Input: dimensioned drawing with shaded views. Units: mm. Origin: part minimum x, y, z. A direction names the side the tool comes from. Coordinates: 2 decimals unless noted, no trailing zeros. Order: outer loops, then holes, each group sorted by start corner. A loop starts at its lowest first (then second) coordinate and runs counter-clockwise, first axis right, second up. Notation, with made-up numbers: (43.25, 83.5) -> (84.25, 83.5) arc R20 ccw to (84.25, 90.5) -> close; hole circle Ø8 at (-12, 13). An arc over 180 degrees is marked (long way). Answer as CSV lines item,"result".
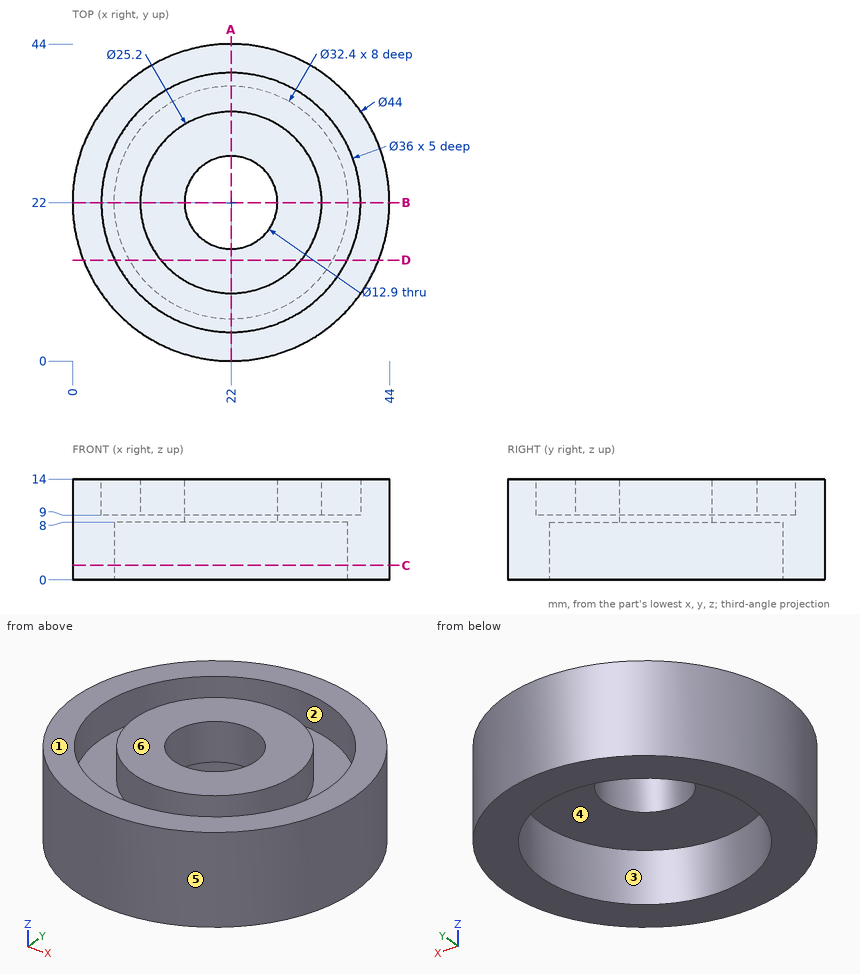
1. Ray query, line 1 along Y through (x, z) = (22, 11.5); line 2 along Y through (x, z) = (22, 6.25); line 3 along X through (y, z) = (13.5, 10.5). Return the intervals inside material, ascending.
Findings:
line 1,"y = 0 to 4, 9.4 to 15.55, 28.45 to 34.6, 40 to 44"
line 2,"y = 0 to 5.8, 38.2 to 44"
line 3,"x = 1.71 to 6.13, 12.7 to 31.3, 37.87 to 42.29"
2. Mould query, pull axis Y, two halves, no side actions, for the marked faces 4, 5 and 6. Classes: released by +Y, released by -Y, zero draft, split by the parting line, or undercut.
Findings:
face 4,"undercut"
face 5,"split by the parting line"
face 6,"zero draft"
3. Contact query for flat-ended pins moving along their axis: pin 1 (6 mm diameter, centred on x = 31.5, y = 31, fed in from +Z); pin 2 (4 mm diameter, centred on y = 34, z = 8.5, fed in from -X); pin 3 (16 mm diameter, centred on x = 22.5, y = 17.5, fed in from -Z); pin 4 (2 mm diameter, centred on x = 34, z = 3.5, fed in from -Y). Output: stop coordinate, or through.
Findings:
pin 1,"stops at z = 14"
pin 2,"stops at x = 2.4"
pin 3,"stops at z = 8"
pin 4,"stops at y = 2.95"
4. Cut plane C-C (z = 2). Return the cut outline in (x, y).
Findings:
outline,"circle Ø44 at (22, 22); hole circle Ø32.4 at (22, 22)"
5. Cut plane A-A (x = 22). Return the cut outline in (y, z), plus the area to 3 significant figures.
Findings:
outline,"(0, 0) -> (5.8, 0) -> (5.8, 8) -> (15.55, 8) -> (15.55, 14) -> (9.4, 14) -> (9.4, 9) -> (4, 9) -> (4, 14) -> (0, 14) -> close; (28.45, 8) -> (38.2, 8) -> (38.2, 0) -> (44, 0) -> (44, 14) -> (40, 14) -> (40, 9) -> (34.6, 9) -> (34.6, 14) -> (28.45, 14) -> close"
area,"225 mm2"
6. Cut plane D-D (y = 14). Return the cut outline in (x, z), plus the area to 3 significant figures.
Findings:
outline,"(1.51, 0) -> (7.91, 0) -> (7.91, 8) -> (36.09, 8) -> (36.09, 0) -> (42.49, 0) -> (42.49, 14) -> (38.12, 14) -> (38.12, 9) -> (31.73, 9) -> (31.73, 14) -> (12.27, 14) -> (12.27, 9) -> (5.88, 9) -> (5.88, 14) -> (1.51, 14) -> close"
area,"285 mm2"
7. Reachability of the marked faces 1, 2 and 3 from +Z, -Z, +X, -X, +Y, -Y: full face, straight path, thin tool, end or side. Return the list, or none.
Findings:
face 1,"+Z, +X, -X, +Y, -Y"
face 2,"+Z"
face 3,"-Z"
